```python
from build123d import *

# Parameters (mm, degrees)
F1_DEPTH = 15
F2_W     = 33
F2_H     = 58
F3_DEPTH = 15.001
F4_W     = 50
F4_H     = 75
F5_DEPTH = 120
F6_R     = 18
F7_DEPTH = 75


# Not quite as in the source:
# - a feature of the source that left no trace in its solid (it failed there, or was rolled back) is left out


with BuildPart() as f1:
    # F0 (on Top) → F1 (new body)
    with BuildSketch(Plane.XY):
        with BuildLine():
            Line((-100, -250), (100, -250))
            ThreePointArc((100, -250), (135.3553390593, -235.3553390593), (150, -200))
            Line((150, -200), (150, 100))
            ThreePointArc((150, 100), (0, 250), (-150, 100))
            Line((-150, 100), (-150, -200))
            ThreePointArc((-150, -200), (-135.3553390593, -235.3553390593), (-100, -250))
        make_face()
    extrude(amount=F1_DEPTH)

    # F2 (on face) → F3 (cut, through all)
    with BuildSketch(Plane.XY.offset(15)):
        with Locations((0, 44)):
            Rectangle(F2_W, F2_H)
    extrude(amount=-F3_DEPTH, mode=Mode.SUBTRACT)

    # F4 (on face) → F5 (join)
    with BuildSketch(Plane.XY.offset(15)):
        with Locations((0, -87.5)):
            Rectangle(F4_W, F4_H)
    extrude(amount=F5_DEPTH)

    # F6 (on face) → F7 (cut, through all)
    with BuildSketch(Plane.XZ.offset(125)):
        with Locations((0, 103.9)):
            Circle(F6_R)
    extrude(amount=-F7_DEPTH, mode=Mode.SUBTRACT)


solid = f1.part
```
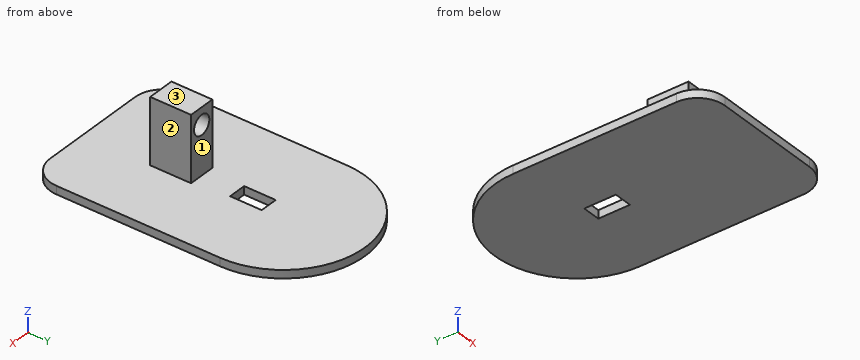
Read the model definition and answer for the solid it produces. Units are mm, in the model's axes. Face numbers are marked on the shaded views. A direction names the side the tool comes from. Give positions to 0.01 mm unless a question says otherwise; leave off trailing zeros. Order: outer loops, then holes, each group sorted by start corner. A loop starts at its lowest first (then second) coordinate and runs counter-clockwise, first axis right, second up.
(1) Find section B-B (z = 103.9). Give the vertices of the cut face in (x, y), plus the area to 3 significant figures.
(2) Given pin 1 (8 mm diameter, centred on x = 40.5, z = 15.5, fed in from +Y); pin 2 (8 mm diameter, centred on x = 52.5, y = -102.5, fed in from +Z); pin 3 (4.5 mm diameter, centred on x = 8, z = 4, fed in from +Y), each flat-ended and moving along its own axis, determine where each tip first touches the part or whether it passes through.
(3) For the marked faces 1, 2 and 3, determine the directions among +Z, -Z, +X, -X, +Y, -Y from which every point of the face is accessible in a straight line to the end or side of a thin tool.
(4) Find section A-A (x = 0). Give the vertices of the cut face in (y, z).
(5) Find section D-D (z = 62.5). Give the vertices of the cut face in (x, y), plus the area to 3 significant figures.
(6) Straight lines are drawn through the part: L1, parallel to Z at x = 0, y = -82; L2, parallel to X at y = 37, z = 14; L3, parallel to X at y = -79, z = 42. For each, find the intervals that lie inside material, in ascending order.
(7) Find section C-C (y = -148.5). Give the vertices of the cut face in (x, z), plus the area to 3 significant figures.
Result sheet:
1. outline: (-25, -125) - (-18, -125) - (-18, -50) - (-25, -50) - close; (18, -125) - (25, -125) - (25, -50) - (18, -50) - close
1. area: 1,050 mm2
2. pin 1: stops at y = 245.48
2. pin 2: stops at z = 15
2. pin 3: stops at y = 249.89
3. face 1: +Z, +X, -X, +Y
3. face 2: +Z, +X, +Y, -Y
3. face 3: +Z, +X, -X, +Y, -Y
4. outline: (-250, 0) - (15, 0) - (15, 15) - (-50, 15) - (-50, 85.9) - (-125, 85.9) - (-125, 15) - (-250, 15) - close; (-125, 121.9) - (-50, 121.9) - (-50, 135) - (-125, 135) - close; (73, 0) - (250, 0) - (250, 15) - (73, 15) - close
5. outline: (-25, -125) - (25, -125) - (25, -50) - (-25, -50) - close
5. area: 3,750 mm2
6. L1: z = 0 to 85.9, 121.9 to 135
6. L2: x = -150 to -16.5, 16.5 to 150
6. L3: x = -25 to 25
7. outline: (-150, 0) - (150, 0) - (150, 15) - (-150, 15) - close
7. area: 4,500 mm2
